Input: part model. Units: mm. Frame: model coordinates. A direction names the side the tool comes from. Coordinates: 2 decimals unless noted, no trailing zeros. Write each loop counter-clockwise with the first axis right and the second up, starting at its lowest first coordinate (ties: lowest second). Pieces come first, ordered by that corner, then holes.
1) Section query A-A (z = -49.5). Output: boundary loops of the cut face in (x, y).
2) Pin query (flat end, axial travel): pin 1 Ø6 at (x, y) = (-12.5, 2) entering from -Z; pin 2 Ø2 at (x, z) = (-0.5, -60.5) entering from -Y; pin 3 Ø5 at (y, z) = (7.5, -21.5) entering from -X; pin 4 Ø4 at (y, z) = (5, -5) entering from -X. Return the tip coordinate at first contact, or that it passes through.
3) Section query D-D (x = -27.5). Output: boundary loops of the cut face in (y, z), then the cut area to 3 significant figures.
4) Section query C-C (y = 7.25). Output: boundary loops of the cut face in (x, z), then the cut area to 3 significant figures.
5) Draft query along Z for faces 3 (the cylindrical face through (1.7, 4.9, -1.5)), 4 (the cylindrical face through (-27, 5, -70)), 5 (the flat face through (0, 5, -17)). Return one class per face: pulls with the +Z half, pulls with the -Z half, needs draft (parallel to the pull), parting line crosses it, or undercut.
6) Section query B-B (z = -32.5). Output: boundary loops of the cut face in (x, y), then the cut area to 3 significant figures.
7) Set-up query: faces 1 (the flat face through (3.5, 5, -7)), 2 (the cylindrical face through (3, 9, -68)). Return all of +Z, -Z, +X, -X, +Y, -Y with unobstructed straight access to the full face (end or side cutting, diameter ignored); none if empty.
8) Line query: L1, parallel to Z at x = 2.75, y = 5; L2, parallel to X at y = 6, z = -52.5; L3, parallel to Y at x = 2.55, z = -5. Output: solid intervals per line, ascending.
from build123d import *
from build123d.topology import SkipClean

# Parameters (mm, degrees)
IZIM1_W                     = 5
IZIM1_H                     = 70
Y_KSEKLIK_EKSTR_ZYON1_DEPTH = 10
IZIM3_R                     = 3.5
KES_EKSTR_ZYON2_DEPTH       = 3.5
IZIM2_R                     = 5
Y_KSEKLIK_EKSTR_ZYON4_DEPTH = 25
RADYUS1_R                   = 5
Y_KSEKLIK_EKSTR_ZYON5_DEPTH = 5


with BuildPart() as part:
    # Çizim1 → Yükseklik-Ekstrüzyon1 (new body)
    with BuildSketch(Plane(origin=(0, 0, 0), x_dir=(1, 0, 0), z_dir=(0, 1, 0))):
        with Locations((2.5, 35)):
            Rectangle(IZIM1_W, IZIM1_H)
    extrude(amount=Y_KSEKLIK_EKSTR_ZYON1_DEPTH)

    # Çizim3 → Kes-Ekstrüzyon2 (cut)
    with BuildSketch(Plane.ZY):
        with Locations((-5, 5)):
            Circle(IZIM3_R)
        with BuildLine():
            ThreePointArc((-5.305535476, 1.513361494), (-8.5, 5), (-5.305535476, 8.486638506))
            Line((-5.305535476, 8.486638506), (-12, 7.9))
            Line((-12, 7.9), (-12, 2.1))
            Line((-12, 2.1), (-5.305535476, 1.513361494))
        make_face()
    extrude(amount=-KES_EKSTR_ZYON2_DEPTH, mode=Mode.SUBTRACT)

    # Çizim2 → Yükseklik-Ekstrüzyon4 (add)
    with BuildSketch(Plane.ZY):
        with Locations(Location((-35, 5, 0), (0, 0, 270))):
            Circle(IZIM2_R)
    extrude(amount=Y_KSEKLIK_EKSTR_ZYON4_DEPTH)

    # Radyus1
    radyus1_edges = [part.edges().sort_by_distance(p)[0] for p in [
        (2.5, 0, -70),
        (2.5, 0, 0),
        (2.5, 10, 0),
        (2.5, 10, -70),
    ]]
    fillet(radyus1_edges, radius=RADYUS1_R - 0.0001)  # a hair under: the kernel refuses the full size

    # Çizim4 → Yükseklik-Ekstrüzyon5 (add)
    with SkipClean():  # the faces are left unmerged after this step: merging them gives an invalid solid
        with BuildSketch(Plane.ZY.offset(25)):
            with BuildLine():
                Line((-35, 0), (-65, 0))
                ThreePointArc((-65, 0), (-70, 5), (-65, 10))
                Line((-65, 10), (-35, 10))
                ThreePointArc((-35, 10), (-30, 5), (-35, 0))
            make_face()
        extrude(amount=Y_KSEKLIK_EKSTR_ZYON5_DEPTH)
    add(part.part.scale(1), mode=Mode.REPLACE)  # the faces are merged on a copy


solid = part.part
Answer:
1. outline: (-30, 0) - (-25, 0) - (-25, 10) - (-30, 10) - close; (0, 0) - (5, 0) - (5, 10) - (0, 10) - close
2. pin 1: stops at z = -40
2. pin 2: stops at y = 0
2. pin 3: stops at x = 0
2. pin 4: stops at x = 3.5
3. outline: (0, -65) arc R5 ccw to (10, -65) - (10, -35) arc R5 ccw to (0, -35) - close
3. area: 379 mm2
4. outline: (-30, -69.47) - (-25, -69.47) - (-25, -39.47) - (0, -39.47) - (0, -69.47) - (5, -69.47) - (5, -0.53) - (0, -0.53) - (0, -2.32) - (3.5, -2.32) - (3.5, -12) - (0, -12) - (0, -30.53) - (-30, -30.53) - close
4. area: 729 mm2
5. face 3: undercut
5. face 4: pulls with the -Z half
5. face 5: needs draft
6. outline: (-30, 0.67) - (0, 0.67) - (0, 0) - (5, 0) - (5, 10) - (0, 10) - (0, 9.33) - (-30, 9.33) - close
6. area: 310 mm2
7. face 1: -X
7. face 2: -Z, +X, -X, +Y
8. L1: z = -70 to -12, -1.5 to 0
8. L2: x = -30 to -25, 0 to 5
8. L3: y = 0 to 1.5, 8.5 to 10
